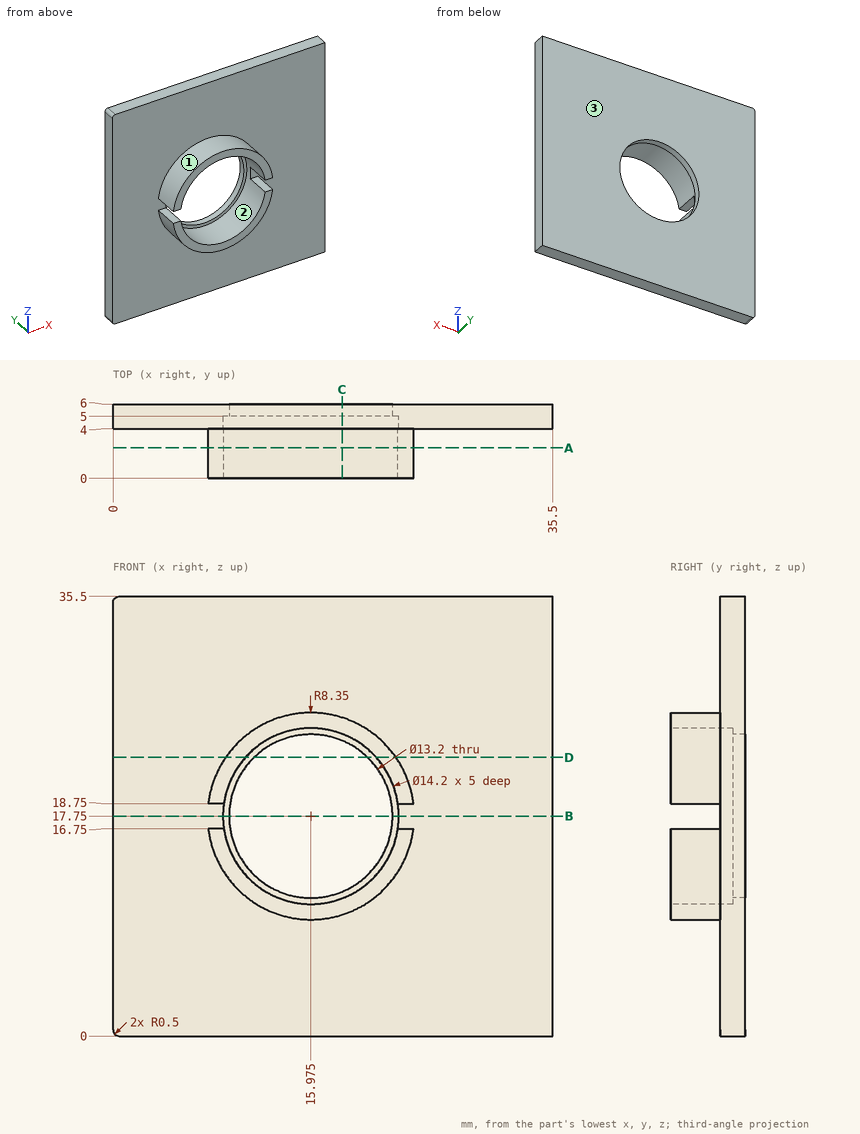
Geometry check sheet. Reference: drawing and pictorial views, mm from the part's lowest x, y, z. Give positions to 0.01 mm unless a question says otherwise; leave off trailing zeros. Write each loop counter-clockwise with the first axis right and the second up, starting at its lowest first coordinate (ties: lowest second). Pieces come first, ordered by that corner, then holes.
Item 1: Cross-section at C-C (x = 18.5). Enter the section's corners in (y, z), and give its area (3 significant figures).
Item 2: Cross-section at A-A (y = 2.45). Enter the section's corners in (x, z) (3 decimals), and give its area (3 significant figures).
Item 3: Scan lines: L1, parallel to Y at x = 23.5, z = 29.5; L2, parallel to X at y = 0.5, z = 23; L3, parallel to X at y = 5.75, z = 13.5. Record each from-to range of solid material in increasing order.
Item 4: Cross-section at D-D (z = 22.5). Enter the section's corners in (x, y), and give its area (3 significant figures).
Item 5: Draft check along Z on the marked faces 1, 2 and 3. Enter one of: released by +Z, released by -Z, zero draft, split by the parting line, or undercut.
Item 6: Gauge pin test, flat ends, axial feed: pin 1 (1.4 mm diameter, centred on x = 8.5, y = 2, fed in from +Z); pin 2 (0.6 mm diameter, centred on x = 8.5, y = 3, fed in from -Z). Record the tip position at first contact, or that the pin passes through.
Item 7: Cross-section at B-B (z = 17.75). Enter the section's corners in (x, y) (3 decimals), and give its area (3 significant figures).
Report:
1. outline: (0, 9.79) - (4, 9.79) - (4, 0) - (6, 0) - (6, 11.65) - (5, 11.65) - (5, 11.11) - (0, 11.11) - close; (0, 24.39) - (5, 24.39) - (5, 23.85) - (6, 23.85) - (6, 35.5) - (4, 35.5) - (4, 25.71) - (0, 25.71) - close
1. area: 56.1 mm2
2. outline: (7.685, 16.75) arc R8.35 ccw to (24.265, 16.75) - (23.004, 16.75) arc R7.1 cw to (8.946, 16.75) - close; (7.685, 18.75) - (8.946, 18.75) arc R7.1 cw to (23.004, 18.75) - (24.265, 18.75) arc R8.35 ccw to start
2. area: 55.7 mm2
3. L1: y = 4 to 6
3. L2: x = 9.48 to 11.2, 20.75 to 22.47
3. L3: x = 0 to 10.93, 21.02 to 35.5
4. outline: (0, 4) - (9.11, 4) - (9.11, 0) - (10.7, 0) - (10.7, 5) - (11.39, 5) - (11.39, 6) - (0, 6) - close; (20.56, 5) - (21.25, 5) - (21.25, 0) - (22.84, 0) - (22.84, 4) - (35.5, 4) - (35.5, 6) - (20.56, 6) - close
4. area: 64.0 mm2
5. face 1: released by +Z
5. face 2: undercut
5. face 3: zero draft
6. pin 1: stops at z = 22.63
6. pin 2: stops at z = 13.48
7. outline: (0, 4) - (8.875, 4) - (8.875, 5) - (9.375, 5) - (9.375, 6) - (0, 6) - close; (22.575, 5) - (23.075, 5) - (23.075, 4) - (35.5, 4) - (35.5, 6) - (22.575, 6) - close
7. area: 43.6 mm2
